from build123d import *

# Parameters (mm, degrees)
CROQUIS1_R              = 75
CROQUIS1_R_2            = 5
CROQUIS1_W              = 24
CROQUIS1_H              = 46.8
CROQUIS1_W_2            = 41.8
CROQUIS1_H_2            = 3.5
CROQUIS1_W_3            = 10
CROQUIS1_H_3            = 10
CROQUIS1_W_4            = 27.8
CROQUIS1_W_5            = 21.5
CROQUIS1_W_6            = 20
CROQUIS1_W_7            = 5
CROQUIS1_H_4            = 11.8
SALIENTE_EXTRUIR1_DEPTH = 3


with BuildPart() as part:
    # Croquis1 → Saliente-Extruir1 (new body)
    with BuildSketch(Plane.XZ):
        with Locations(Location((-2.614604162, 2.776770239, 0), (0, 0, 270))):
            Circle(CROQUIS1_R)
        with Locations(Location((-2.546416873, 39.226770239, 0), (0, 0, 270))):
            Circle(CROQUIS1_R_2, mode=Mode.SUBTRACT)
        with Locations((49.385395838, 2.776770239)):
            Rectangle(CROQUIS1_W, CROQUIS1_H, mode=Mode.SUBTRACT)
        with Locations((-54.614604162, 2.776770239)):
            Rectangle(CROQUIS1_W, CROQUIS1_H, mode=Mode.SUBTRACT)
        with Locations((-2.614604162, -54.673229761)):
            Rectangle(CROQUIS1_W_2, CROQUIS1_H_2, mode=Mode.SUBTRACT)
        with Locations((21.685395838, 10.676770239)):
            Rectangle(CROQUIS1_W_3, CROQUIS1_H_3, mode=Mode.SUBTRACT)
        with Locations((21.685395838, -5.123229761)):
            Rectangle(CROQUIS1_W_3, CROQUIS1_H_3, mode=Mode.SUBTRACT)
        with Locations((-28.114604162, 10.676770239)):
            Rectangle(CROQUIS1_W_3, CROQUIS1_H_3, mode=Mode.SUBTRACT)
        with Locations((-28.114604162, -5.123229761)):
            Rectangle(CROQUIS1_W_3, CROQUIS1_H_3, mode=Mode.SUBTRACT)
        with Locations((19.785395838, 46.226770239)):
            Rectangle(CROQUIS1_W_4, CROQUIS1_H_2, mode=Mode.SUBTRACT)
        with Locations((19.785395838, 39.226770239)):
            Rectangle(CROQUIS1_W_4, CROQUIS1_H_2, mode=Mode.SUBTRACT)
        with Locations((-25.014604162, 46.226770239)):
            Rectangle(CROQUIS1_W_4, CROQUIS1_H_2, mode=Mode.SUBTRACT)
        with Locations((-25.014604162, 39.226770239)):
            Rectangle(CROQUIS1_W_4, CROQUIS1_H_2, mode=Mode.SUBTRACT)
        with Locations((19.785395838, -33.673229761)):
            Rectangle(CROQUIS1_W_4, CROQUIS1_H_2, mode=Mode.SUBTRACT)
        with Locations((19.785395838, -40.673229761)):
            Rectangle(CROQUIS1_W_4, CROQUIS1_H_2, mode=Mode.SUBTRACT)
        with Locations((-25.014604162, -33.673229761)):
            Rectangle(CROQUIS1_W_4, CROQUIS1_H_2, mode=Mode.SUBTRACT)
        with Locations((-25.014604162, -40.673229761)):
            Rectangle(CROQUIS1_W_4, CROQUIS1_H_2, mode=Mode.SUBTRACT)
        with Locations((-20.364604162, 32.226770239)):
            Rectangle(CROQUIS1_W_5, CROQUIS1_H_2, mode=Mode.SUBTRACT)
        with Locations((16.635395838, 53.226770239)):
            Rectangle(CROQUIS1_W_5, CROQUIS1_H_2, mode=Mode.SUBTRACT)
        with Locations((15.135395838, 32.226770239)):
            Rectangle(CROQUIS1_W_5, CROQUIS1_H_2, mode=Mode.SUBTRACT)
        with Locations((-21.864604162, 53.226770239)):
            Rectangle(CROQUIS1_W_5, CROQUIS1_H_2, mode=Mode.SUBTRACT)
        with Locations((16.635395838, -47.673229761)):
            Rectangle(CROQUIS1_W_5, CROQUIS1_H_2, mode=Mode.SUBTRACT)
        with Locations((-21.864604162, -47.673229761)):
            Rectangle(CROQUIS1_W_5, CROQUIS1_H_2, mode=Mode.SUBTRACT)
        with Locations((15.885395838, -26.673229761)):
            Rectangle(CROQUIS1_W_6, CROQUIS1_H_2, mode=Mode.SUBTRACT)
        with Locations((-21.114604162, -26.673229761)):
            Rectangle(CROQUIS1_W_6, CROQUIS1_H_2, mode=Mode.SUBTRACT)
        with Locations((7.185395838, 2.776770239)):
            Rectangle(CROQUIS1_W_7, CROQUIS1_H_4, mode=Mode.SUBTRACT)
        with Locations((-13.614604162, 2.776770239)):
            Rectangle(CROQUIS1_W_7, CROQUIS1_H_4, mode=Mode.SUBTRACT)
    extrude(amount=-SALIENTE_EXTRUIR1_DEPTH)


solid = part.part
Could you check a few things on this model? Use its own coordinates, in mm. Give positions to 0.01 mm unless a question says otherwise; leave off trailing zeros. Loops run counter-clockwise (first coordinate to the right, second up) from the corner with the lowest first, then second, coordinate; pieces in that order, holes last. Notation, with made-up numbers: M 10,-17 L 58,-17 A3 ccw 58,-13 Z; hole C -30.5,35 d4. An arc over 180 degrees is marked long. Answer as a JSON object with one key per item and string values.
Q1. For P1, Ø1.5, axis at x = -27, y = 1.5, coming from the -Z side; P2, Ø1.5, axis at x = -21.5, y = 1, coming from the +Z side; P3, Ø1.5, axis at y = 1.5, z = 32.5, coming from the -X side, each with a flat end and sliding along its axis, tell me the tip position at first contact or that it passes through.
Values found:
{"P1": "stops at z = -68.4", "P2": "stops at z = 75.55", "P3": "stops at x = -71.79"}
Q2. If I drill on probe 1 along X at (y, z) = (2.1, 52.5); probe 2 along X at (y, z) = (2, 11.5); probe 3 along X at (y, z) = (2.5, -7), over which ranges is the centre line in solid material (lowest first)? Write a range as [from, to].
Values found:
{"probe 1": "x = [-58.76, -32.61], [-11.11, 5.89], [27.39, 53.53]", "probe 2": "x = [-77.11, -66.61], [-42.61, -33.11], [-23.11, 16.69], [26.69, 37.39], [61.39, 71.88]", "probe 3": "x = [-76.97, -66.61], [-42.61, -33.11], [-23.11, 16.69], [26.69, 37.39], [61.39, 71.75]"}
Q3. Suppose I cut it at C-C, the plane z = 3. List the corners of the cut face in (x, y) for me, plus the area to 3 significant figures.
Values found:
{"outline": "M -77.61,0 L -66.61,0 L -66.61,3 L -77.61,3 Z; M -42.61,0 L -16.11,0 L -16.11,3 L -42.61,3 Z; M -11.11,0 L 4.69,0 L 4.69,3 L -11.11,3 Z; M 9.69,0 L 37.39,0 L 37.39,3 L 9.69,3 Z; M 61.39,0 L 72.39,0 L 72.39,3 L 61.39,3 Z", "area": "276 mm²"}
Q4. Suppose I cut it at A-A, the plane z = -14.5. List the corners of the cut face in (x, y) for me, plus the area to 3 significant figures.
Values found:
{"outline": "M -75.6,0 L -66.61,0 L -66.61,3 L -75.6,3 Z; M -42.61,0 L 37.39,0 L 37.39,3 L -42.61,3 Z; M 61.39,0 L 70.37,0 L 70.37,3 L 61.39,3 Z", "area": "294 mm²"}
Q5. Suppose I cut it at D-D, the plane x = -49.5. List the corners of the cut face in (y, z) for me.
Values found:
{"outline": "M 0,-55.76 L 3,-55.76 L 3,-20.62 L 0,-20.62 Z; M 0,26.18 L 3,26.18 L 3,61.32 L 0,61.32 Z"}
Q6. Suppose I cut it at B-B, the plane x = 54. List the corners of the cut face in (y, z) for me, plus the area to 3 significant figures.
Values found:
{"outline": "M 0,-46.41 L 3,-46.41 L 3,-20.62 L 0,-20.62 Z; M 0,26.18 L 3,26.18 L 3,51.97 L 0,51.97 Z", "area": "155 mm²"}
